Work out the finished part from the listing and answer in its coordinate system (mm). Face numbers are marked on the shaded views. A direction names the side the tool comes from. Round coordinates to 2 decimals unless told otherwise and drop trailing zeros. Order: outer loops, then holes, each group sorted by start corner. A loop starts at its lowest first (then second) coordinate and runs counter-clockwise, first axis right, second up. Notation, with made-up numbers: (14.5, 54.25) -> (73.5, 54.25) arc R19 ccw to (73.5, 63.25) -> close; hole circle Ø7 at (39, 81). An arc over 180 degrees is marked (long way). Use a Markdown table: item, result. Add a question column.
Item 1: A cutting plane is placed at A-A, the plane z = 0. Determine the outline of the cut face in (x, y), plus the area to 3 significant figures.
Item 2: A tool of negligible diameter and unlimited length cuts with its end or side. For the marked faces 1, 2, 3 and 4, from which of +Z, -Z, +X, -X, +Y, -Y can it reach the whole face along a straight path? Write none if from no direction.
Item 3: Find the intervals of material crossed by L1, parallel to X at y = 71, z = -0.25; L2, parallel to Y at x = 2.5, z = -5.5; L3, parallel to X at y = 57.5, z = 7, in increasing order. Write a range as [from, to].
Item 4: Flat-ended cylindrical pins translate along their axes: P1, Ø6, axis at x = 3.5, z = -5.5, coming from the -Y side; P2, Ø8, axis at x = 0, y = 3, coming from the -Z side; P3, Ø4, axis at y = 40, z = 2.5, coming from the +X side; P4, Ø4, axis at x = -5.5, y = 92.5, coming from the -Z side. Find the tip coordinate at first contact, or state that the pin passes through.
Item 5: A cutting plane is placed at B-B, the plane y = 59. Determine the outline of the cut face in (x, z), plus the area to 3 significant figures.
Item 6: A cutting plane is placed at C-C, the plane y = 7. Determine the outline of the cut face in (x, z).
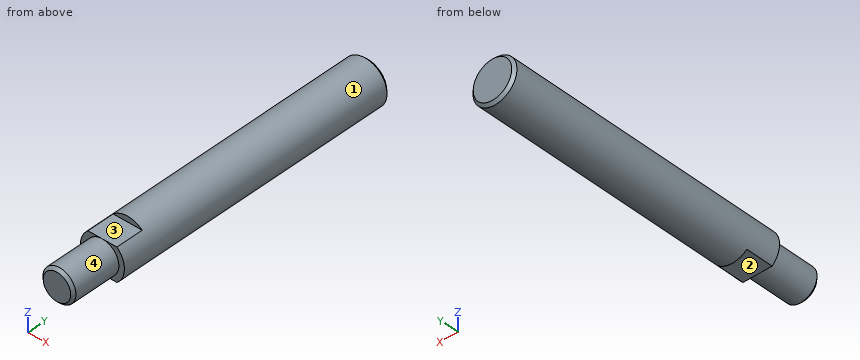
from build123d import *

# Parameters (mm, degrees)
ESBO_O1_R                = 8
RESSALTO_EXTRUS_O1_DEPTH = 105
ESBO_O2_R                = 6
RESSALTO_EXTRUS_O2_DEPTH = 18
CHANFRO1_SIZE            = 1
ESBO_O3_OUTSIDE_W        = 43.012
ESBO_O3_OUTSIDE_H        = 43.012
CORTE_EXTRUS_O1_DEPTH    = 10


with BuildPart() as part:
    # Esboço1 → Ressalto-extrusão1 (new body)
    with BuildSketch(Plane(origin=(0, 0, 0), x_dir=(1, 0, 0), z_dir=(0, 1, 0))):
        with Locations(Location((0, 0, 0), (0, 0, 270))):  # turned: the seam where the file's is
            Circle(ESBO_O1_R)
    extrude(amount=RESSALTO_EXTRUS_O1_DEPTH)

    # Esboço2 → Ressalto-extrusão2 (add)
    with BuildSketch(Plane.XZ):
        with Locations(Location((0, 0, 0), (0, 0, 270))):  # turned: the seam where the file's is
            Circle(ESBO_O2_R)
    extrude(amount=RESSALTO_EXTRUS_O2_DEPTH)

    # Chanfro1
    chanfro1_edges = [part.edges().sort_by_distance(p)[0] for p in [
        (0, 105, -8),
        (0, -18, 6),
    ]]
    chamfer(chanfro1_edges, length=CHANFRO1_SIZE)

    # Esboço3 outside → Corte-extrusão1 (cut)
    with BuildSketch(Plane.XZ):
        Rectangle(ESBO_O3_OUTSIDE_W, ESBO_O3_OUTSIDE_H)
        with BuildLine():
            Line((-8, 6), (8, 6))
            ThreePointArc((8, 6), (14, 0), (8, -6))
            Line((8, -6), (-8, -6))
            ThreePointArc((-8, -6), (-14, 0), (-8, 6))
        make_face(mode=Mode.SUBTRACT)
    extrude(amount=-CORTE_EXTRUS_O1_DEPTH, mode=Mode.SUBTRACT)


solid = part.part
Reported:
| question | item | result |
|---|---|---|
| 1 | outline | (-8, 0) -> (-6, 0) -> (-6, -17) -> (-5, -18) -> (5, -18) -> (6, -17) -> (6, 0) -> (8, 0) -> (8, 104) -> (7, 105) -> (-7, 105) -> (-8, 104) -> close |
| 1 | area | 1,890 mm² |
| 2 | face 1 | +Y, -Y |
| 2 | face 2 | -Z, +X, -X, -Y |
| 2 | face 3 | +Z, +X, -X, -Y |
| 2 | face 4 | -Y |
| 3 | L1 | [-8, 8] |
| 3 | L2 | [0, 105] |
| 3 | L3 | [-3.87, 3.87] |
| 4 | P1 | y = -18 |
| 4 | P2 | z = -6 |
| 4 | P3 | x = 7.98 |
| 4 | P4 | z = -7.19 |
| 5 | outline | circle Ø16 at (0, 0) |
| 5 | area | 201 mm² |
| 6 | outline | (-5.29, -6) -> (5.29, -6) arc R8 ccw to (5.29, 6) -> (-5.29, 6) arc R8 ccw to start |
